Read the model definition and answer for the solid it produces. Units are mm, in the model's axes. Coordinates: 2 decimals unless noted, no trailing zeros. Loops run counter-clockwise (first coordinate to the right, second up) from the corner with the lowest first, then second, coordinate; pieces in that order, holes last. Notation, with made-up numbers: (-40, 80.25) - (-27, 80.25) arc R27 cw to (-27, 117.25) - close; hole circle Ø2 at (51, -22.75). An arc over 180 degrees is marked (long way). Use CSV: the item, a comma, the result in double quotes.
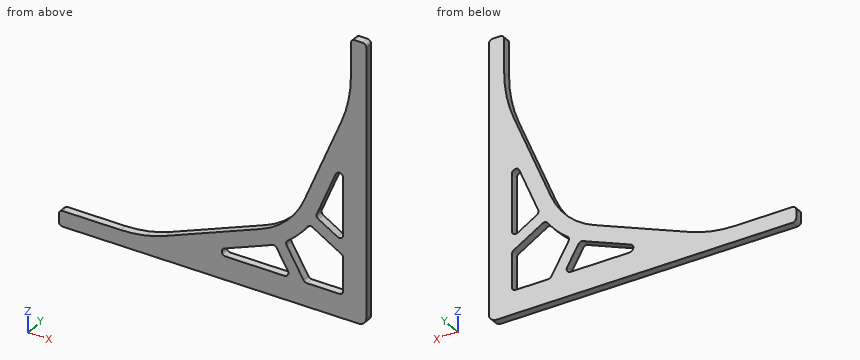
```python
from build123d import *

# Parameters (mm, degrees)
F1_DEPTH = 6.35
F2_R     = 3.175


with BuildPart() as f1:
    # F0 (on Front) → F1 (new body)
    with BuildSketch(Plane.XZ):
        with BuildLine():
            Line((-254, 12.7), (-254, 0))
            Line((-254, 0), (-6.35, 0))
            ThreePointArc((-6.35, 0), (-1.859872, 1.859872), (0, 6.35))
            Line((0, 6.35), (0, 228.6))
            Line((0, 228.6), (-12.7, 228.6))
            Line((-12.7, 228.6), (-12.7, 198.205883))
            ThreePointArc((-12.7, 198.205883), (-14.689229, 178.199527), (-20.579021, 158.976581))
            Line((-20.579021, 158.976581), (-51.366437, 85.423735))
            ThreePointArc((-51.366437, 85.423735), (-65.554229, 64.533113), (-86.762078, 50.82404))
            Line((-86.762078, 50.82404), (-166.112046, 19.711186))
            ThreePointArc((-166.112046, 19.711186), (-184.327579, 14.468183), (-203.2, 12.7))
            Line((-203.2, 12.7), (-254, 12.7))
        make_face()
        with BuildLine():
            Line((-117.371321, 25.1809), (-82.126084, 39.000439))
            ThreePointArc((-82.126084, 39.000439), (-80.06592, 39.843141), (-78.031249, 40.745656))
            ThreePointArc((-78.031249, 40.745656), (-75.753604, 40.892633), (-73.965863, 39.473743))
            Line((-73.965863, 39.473743), (-64.755951, 23.83627))
            ThreePointArc((-64.755951, 23.83627), (-64.735236, 20.64943), (-67.49172, 19.05))
            Line((-67.49172, 19.05), (-116.212322, 19.05))
            ThreePointArc((-116.212322, 19.05), (-119.332067, 21.635237), (-117.371321, 25.1809))
        make_face(mode=Mode.SUBTRACT)
        with BuildLine():
            Line((-51.80374, 20.61373), (-65.758555, 44.307554))
            ThreePointArc((-65.758555, 44.307554), (-66.132559, 46.559084), (-64.899556, 48.479753))
            ThreePointArc((-64.899556, 48.479753), (-56.060512, 56.060512), (-48.479753, 64.899556))
            ThreePointArc((-48.479753, 64.899556), (-46.559084, 66.132559), (-44.307554, 65.758555))
            Line((-44.307554, 65.758555), (-20.61373, 51.80374))
            ThreePointArc((-20.61373, 51.80374), (-19.468516, 50.643541), (-19.05, 49.067971))
            Line((-19.05, 49.067971), (-19.05, 22.225))
            ThreePointArc((-19.05, 22.225), (-19.979936, 19.979936), (-22.225, 19.05))
            Line((-22.225, 19.05), (-49.067971, 19.05))
            ThreePointArc((-49.067971, 19.05), (-50.643541, 19.468516), (-51.80374, 20.61373))
        make_face(mode=Mode.SUBTRACT)
        with BuildLine():
            Line((-39.651315, 80.520073), (-25.153781, 115.155487))
            ThreePointArc((-25.153781, 115.155487), (-21.599801, 117.042408), (-19.05, 113.929571))
            Line((-19.05, 113.929571), (-19.05, 67.49172))
            ThreePointArc((-19.05, 67.49172), (-20.64943, 64.735236), (-23.83627, 64.755951))
            Line((-23.83627, 64.755951), (-39.473743, 73.965863))
            ThreePointArc((-39.473743, 73.965863), (-40.892633, 75.753604), (-40.745656, 78.031249))
            ThreePointArc((-40.745656, 78.031249), (-40.187384, 79.27078), (-39.651315, 80.520073))
        make_face(mode=Mode.SUBTRACT)
    extrude(amount=F1_DEPTH)

    # F2
    f2_edges = [f1.edges().sort_by_distance(p)[0] for p in [
        (-254, -3.175, 0),
        (-254, -3.175, 12.7),
        (0, -3.175, 228.6),
        (-12.7, -3.175, 228.6),
    ]]
    fillet(f2_edges, radius=F2_R)


solid = f1.part
```
Q1. The part is cut by section D-D on z = 153.5. Determine the outline of the cut face in (x, y).
Reported:
outline,"(-22.87, -6.35) - (0, -6.35) - (0, 0) - (-22.87, 0) - close"
Q2. The part is cut by section B-B on y = -2.5. Give the number of separate pieces and of enclosed holes in the cut face, and give its area (3 significant figures).
Reported:
separate pieces,"1"
enclosed holes,"3"
area,"11,100 mm²"
Q3. The part is cut by section A-A on x = -109. Determine the outline of the cut face in (y, z).
Reported:
outline,"(-6.35, 0) - (0, 0) - (0, 19.05) - (-6.35, 19.05) - close; (-6.35, 28.46) - (0, 28.46) - (0, 42.1) - (-6.35, 42.1) - close"
Q4. Find the intervals of material crossed by probe 1 along Z at (x, y) = (-30, -1); probe 2 along Z at (x, y) = (-213, -2); probe 3 along X at (y, z) = (-1, 67), in increasing order. Write a range as [from, to].
Reported:
probe 1,"z = [0, 19.05], [57.33, 68.39], [103.58, 136.47]"
probe 2,"z = [0, 12.7]"
probe 3,"x = [-63.16, -27.65], [-19.09, 0]"
Q5. The part is cut by section C-C on x = -213. Determine the outline of the cut face in (y, z), and give its area (3 significant figures).
Reported:
outline,"(-6.35, 0) - (0, 0) - (0, 12.7) - (-6.35, 12.7) - close"
area,"80.6 mm²"
Q6. Given P1, Ø3, axis at y = -2.5, z = 88, coming from the -X side; P2, Ø1, axis at x = -142.5, y = -1.5, coming from the +Z side; P3, Ø1.9, axis at x = -85, y = -4.5, coming from the +Z side, each flat-ended and moving along its own axis, determine where each tip first touches the part or whether it passes through.
Reported:
P1,"stops at x = -50.92"
P2,"stops at z = 29.17"
P3,"stops at z = 51.96"
